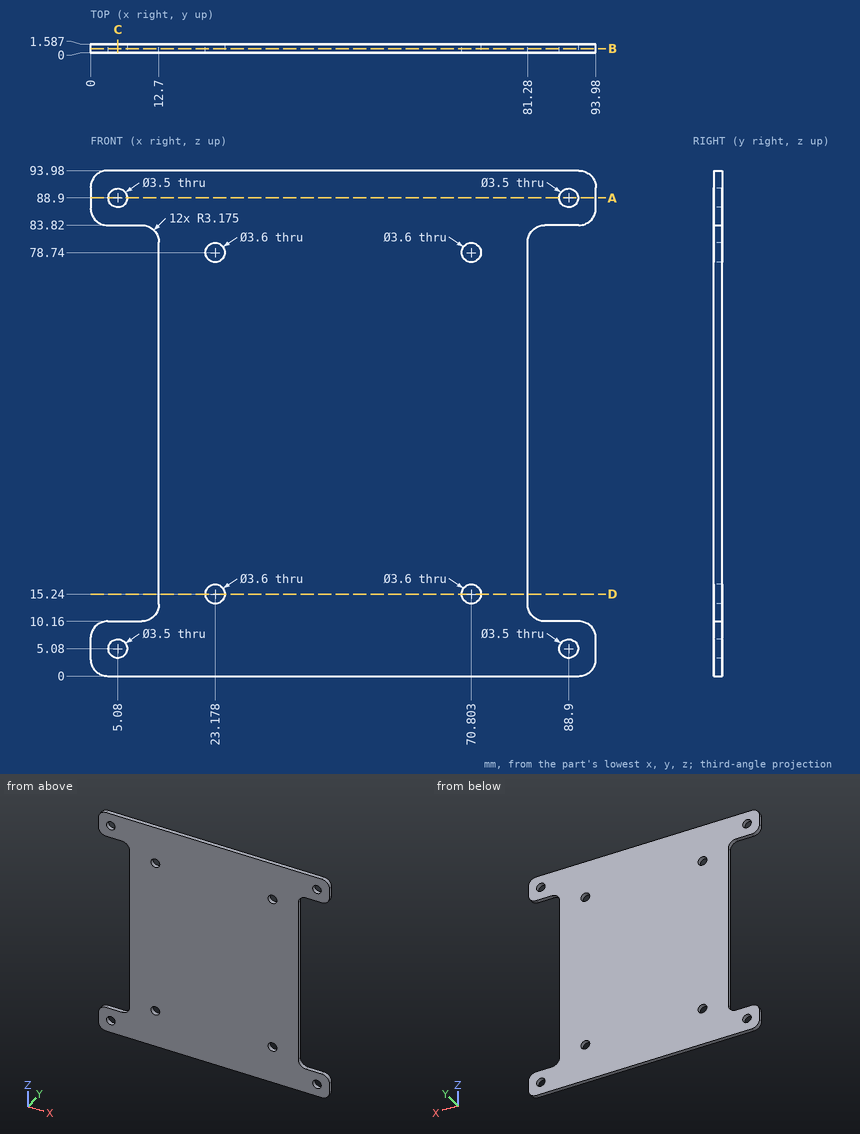
Can you work these out from the drawing? Everything is in mm from the part's minimum corner. Coordinates: 2 decimals unless noted, no trailing zeros. Order: outer loops, then holes, each group sorted by start corner. A loop starts at its lowest first (then second) coordinate and runs counter-clockwise, first axis right, second up. Notation, with made-up numbers: (8.5, 63.25) -> (35.5, 63.25) arc R26 cw to (35.5, 83.25) -> close; hole circle Ø5 at (-5.75, -14). An arc over 180 degrees is marked (long way). Return JSON: item names as keys, results as strings.
1) If we section it at D-D on z = 15.24: List the corners of the cut face in (x, y) for me.
Conclusion:
{"outline": "(12.7, 0) -> (21.38, 0) -> (21.38, 1.59) -> (12.7, 1.59) -> close; (24.98, 0) -> (69, 0) -> (69, 1.59) -> (24.98, 1.59) -> close; (72.6, 0) -> (81.28, 0) -> (81.28, 1.59) -> (72.6, 1.59) -> close"}
2) If we section it at A-A on z = 88.9: List the corners of the cut face in (x, y) for me.
Conclusion:
{"outline": "(0, 0) -> (3.33, 0) -> (3.33, 1.59) -> (0, 1.59) -> close; (6.83, 0) -> (87.15, 0) -> (87.15, 1.59) -> (6.83, 1.59) -> close; (90.65, 0) -> (93.98, 0) -> (93.98, 1.59) -> (90.65, 1.59) -> close"}
3) If I drill on probe 1 along Z at (x, y) = (88.9, 1.2); probe 2 along X at (y, z) = (1.2, 88.9); probe 3 along Z at (x, y) = (87.5, 0.15), over which ranges is the centre line in solid material (lowest first)?
Conclusion:
{"probe 1": "z = 0 to 3.33, 6.83 to 10.16, 83.82 to 87.15, 90.65 to 93.98", "probe 2": "x = 0 to 3.33, 6.83 to 87.15, 90.65 to 93.98", "probe 3": "z = 0 to 4.03, 6.13 to 10.16, 83.82 to 87.85, 89.95 to 93.98"}
4) If we section it at C-C on x = 5.08: List the corners of the cut face in (y, z) for me.
Conclusion:
{"outline": "(0, 0) -> (1.59, 0) -> (1.59, 3.33) -> (0, 3.33) -> close; (0, 6.83) -> (1.59, 6.83) -> (1.59, 10.16) -> (0, 10.16) -> close; (0, 83.82) -> (1.59, 83.82) -> (1.59, 87.15) -> (0, 87.15) -> close; (0, 90.65) -> (1.59, 90.65) -> (1.59, 93.98) -> (0, 93.98) -> close"}
5) If we section it at B-B on y = 0.75: State how many separate pieces and enclosed holes the cut face has, plus the area to 3 significant figures.
Conclusion:
{"separate pieces": "1", "enclosed holes": "8", "area": "6,870 mm²"}
6) I'm going to push flat-ended pins straight in: P1, Ø3, axis at x = 70.8, z = 15.24, coming from the +Y side; P2, Ø4.5, axis at x = 88.9, z = 88.9, coming from the +Y side; P3, Ø0.5, axis at y = 1, z = 57.5, coming from the +X side; P4, Ø0.5, axis at y = 0.5, z = 47.5, coming from the -X side. Where does each tip first touch, or does it pass through?
Conclusion:
{"P1": "passes through", "P2": "stops at y = 1.59", "P3": "stops at x = 81.28", "P4": "stops at x = 12.7"}
